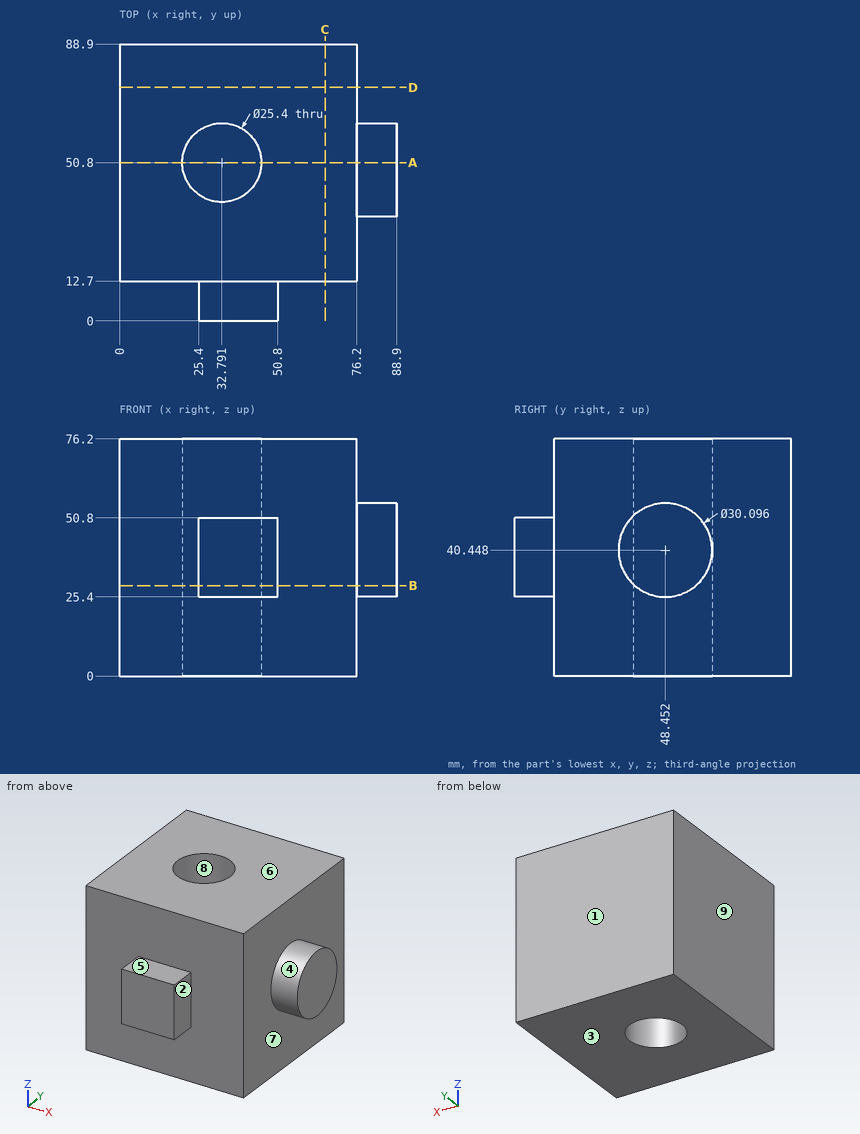
Input: dimensioned drawing with shaded views. Units: mm. Origin: part minimum x, y, z. A direction names the side the tool comes from. Give positions to 0.01 mm unless a question says otherwise; leave off trailing zeros. Write each loop counter-clockwise with the first axis right and the second up, starting at its lowest first coordinate (ties: lowest second). Pieces come first, ordered by that corner, then holes.
1. Section query B-B (z = 29). Return the cut outline in (x, y) (1 decimal), then the cut area to 3 significant figures.
2. Material intervals for line 1 along X through (y, z) = (50, 20); line 2 along X through (y, z) = (50, 45); line 3 along Y through (x, z) = (32, 43.5) (1 decimal), sorted ascending.
3. First-contact query: pin 1 (6.5 mm diameter, centred on y = 4.5, z = 38.5, fed in from -X); pin 2 (14 mm diameter, centred on y = 5, z = 35, fed in from +X); pin 3 (12 mm diameter, centred on y = 15.5, z = 13, fed in from +X); pin 4 (12 mm diameter, centred on x = 26.5, y = 50, fed in from +Z). Flat tips, straight axial feed; report the tip coordinate or a pass-through.
4. Section query C-C (x = 66). Return the cut outline in (y, z), then the cut area to 3 significant figures.
5. Pull-direction query (X, two-part tool) for the marked faces 6, 7, 8 and 9; classes: +X half, -X half, draft (parallel to the pull), parting line (faces both ways), or undercut.
6. Section query A-A (y = 50.8). Return the cut outline in (x, z), then the cut area to 3 significant figures.
7. Section query D-D (y = 75). Return the cut outline in (x, z), then the cut area to 3 significant figures.
8. Access query for the marked faces 1, 2, 3, 4 and 5. Directions: +Z, -Z, +X, -X, +Y, -Y. A direction counts if a zero-diameter tool reaches every point of the face in a straight line with its end or side. Return the directions, or none.
Output values:
1. outline: (0, 12.7) - (25.4, 12.7) - (25.4, 0) - (50.8, 0) - (50.8, 12.7) - (76.2, 12.7) - (76.2, 38.7) - (88.9, 38.7) - (88.9, 58.2) - (76.2, 58.2) - (76.2, 88.9) - (0, 88.9) - close; hole circle Ø25.4 at (32.8, 50.8)
1. area: 5,870 mm2
2. line 1: x = 0 to 20.12, 45.47 to 76.2
2. line 2: x = 0 to 20.12, 45.47 to 88.9
2. line 3: y = 0 to 38.1, 63.5 to 88.9
3. pin 1: stops at x = 25.4
3. pin 2: stops at x = 50.8
3. pin 3: stops at x = 76.2
3. pin 4: passes through
4. outline: (12.7, 0) - (88.9, 0) - (88.9, 76.2) - (12.7, 76.2) - close
4. area: 5,810 mm2
5. face 6: draft
5. face 7: +X half
5. face 8: undercut
5. face 9: -X half
6. outline: (0, 0) - (20.09, 0) - (20.09, 76.2) - (0, 76.2) - close; (45.49, 0) - (76.2, 0) - (76.2, 25.58) - (88.9, 25.58) - (88.9, 55.31) - (76.2, 55.31) - (76.2, 76.2) - (45.49, 76.2) - close
6. area: 4,250 mm2
7. outline: (0, 0) - (76.2, 0) - (76.2, 76.2) - (0, 76.2) - close
7. area: 5,810 mm2
8. face 1: +Z, -Z, +X, -X, +Y
8. face 2: +Z, -Z, +X, -Y
8. face 3: -Z, +X, -X, +Y, -Y
8. face 4: +X
8. face 5: +Z, +X, -X, -Y
